```python
from build123d import *

# Parameters (mm, degrees)
BOSS_EXTRUDE1_DEPTH = 35
CUT_EXTRUDE2_DEPTH  = 10
CUT_EXTRUDE3_DEPTH  = 35
SKETCH7_W           = 1.915857316
SKETCH7_H           = 33.660559038
CUT_EXTRUDE4_DEPTH  = 0.1


with BuildPart() as part:
    # Sketch1 → Revolve1 (revolve)
    with BuildSketch(Plane.XY, mode=Mode.PRIVATE) as revolve1_sk:
        Polygon((373.098534333, 35.069747422), (349.598534333, 35.069747422), (349.598534333, 36.051468212), (373.098534333, 36.051468212), (400.761964989, 66.939755158), (401.975618585, 66.939755158), align=None)
    revolve(revolve1_sk.sketch.rotate(Axis((349.598534333, 66.939755158, 0), (0, -1, 0)), 90), axis=Axis((349.598534333, 66.939755158, 0), (0, -1, 0)))

    # Sketch2 → Boss-Extrude1 (add)
    with BuildSketch(Plane(origin=(0, 66.939755158, 0), x_dir=(1, 0, 0), z_dir=(0, 1, 0))):
        with BuildLine():
            ThreePointArc((351.491870795, 51.128386573), (349.575661264, 51.163425543), (347.659483828, 51.12667327))
            Line((347.659483828, 51.12667327), (345.790974227, -51.02155547))
            ThreePointArc((345.790974227, -51.02155547), (347.704525671, -51.128361676), (349.620734741, -51.16342584))
            Line((349.620734741, -51.16342584), (351.491870795, 51.128386573))
        make_face()
    extrude(amount=-BOSS_EXTRUDE1_DEPTH)

    # Sketch3 → Cut-Extrude2 (cut)
    with BuildSketch(Plane(origin=(350.439365404, 0, 6.410285591), x_dir=(0.018289079495206917, 0, -0.9998327407977887), z_dir=(0.9998327407977886, 0, 0.018289079495206913))):
        Polygon((-44.760626875, 65.600314196), (-17.086632512, 35.069747422), (29.874303283, 35.069747422), (57.548297647, 65.600314196), (57.842029456, 31.939755158), (-44.760626875, 31.939755158), align=None)
    extrude(amount=-CUT_EXTRUDE2_DEPTH, mode=Mode.SUBTRACT)

    # Sketch6 → Cut-Extrude3 (cut)
    with BuildSketch(Plane(origin=(0, 66.939755158, 0), x_dir=(1, 0, 0), z_dir=(0, 1, 0))):
        Polygon((350.109498728, -52.374591838), (349.598534333, -52.377084252), (349.598534333, -53.887685529), (342.379231724, -53.887685529), (345.988883028, -52.252553739), align=None)
    extrude(amount=-CUT_EXTRUDE3_DEPTH, mode=Mode.SUBTRACT)


with BuildPart() as cut_extrude3_kept_piece:
    # of the separate pieces the step leaves, the one the design keeps (cut_extrude3_pieces_kept)
    add(part.part.solids().sort_by_distance((350.985738912, 35.069747422, -23.45902094))[0])

    # Sketch7 → Cut-Extrude4 (cut)
    with BuildSketch(Plane(origin=(-0.818630663, 0, 44.753140248), x_dir=(-0.9998327407977887, 0, -0.01828907949520692), z_dir=(0.018289079495206917, 0, -0.9998327407977886))):
        with Locations((-349.540060761, 48.770034677)):
            Rectangle(SKETCH7_W, SKETCH7_H)
    extrude(amount=-CUT_EXTRUDE4_DEPTH, mode=Mode.SUBTRACT)


solid = cut_extrude3_kept_piece.part
```
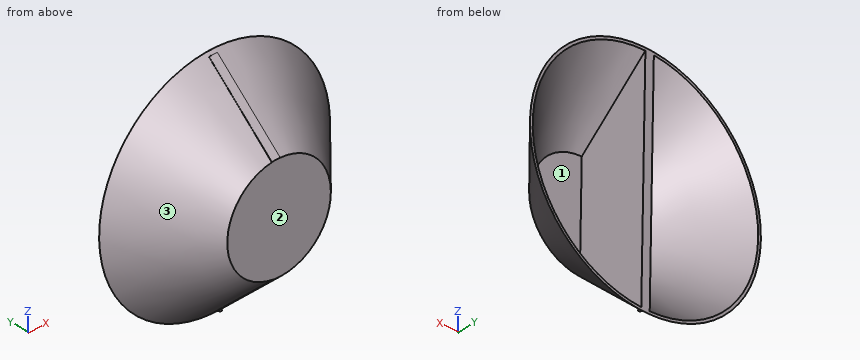
Model file for the job. Use its own axes, mm. Face numbers are marked on the shaded views. Round coordinates to 2 decimals unless told otherwise and drop trailing zeros. Write each loop counter-clockwise with the first axis right and the second up, starting at its lowest first coordinate (ties: lowest second). Pieces come first, ordered by that corner, then holes. Notation, with made-up numbers: (-18, 62.25) - (-8, 62.25) arc R10 cw to (-8, 78.25) - close; hole circle Ø3 at (44, -1.75). An arc over 180 degrees is marked (long way). One line per item, written item: value.
(1) Drop flat-ended pins along their axis: P1, Ø10, axis at x = 374, z = -17, coming from the +Y side; P2, Ø1, axis at x = 378, y = 62, coming from the -Z side; P3, Ø5, axis at x = 372.5, z = 32, coming from the +Y side. Give the stop position or say it passes through.
Values follow:
P1: stops at y = 48.6
P2: stops at z = -39.24
P3: stops at y = 56.54
(2) Cut at B-B, the plane z = 0. Give the cut face in (x, y).
Values follow:
outline: (297.22, 66.94) - (326.1, 35.07) - (373.1, 35.07) - (401.98, 66.94) - (400.76, 66.94) - (373.1, 36.05) - (350.56, 36.05) - (350.56, 66.94) - (346.72, 66.94) - (346.72, 36.05) - (326.1, 36.05) - (298.44, 66.94) - close
(3) Wall check: probe 1 along X at (y, z) = (59.5, 24); probe 2 along X at (y, z) = (38, 6.5); probe 3 along Z at (x, y) = (371, 62.5). Give the ranges that are in metal, low to high.
Values follow:
probe 1: x = 310.78 to 312.12, 346.29 to 350.12, 387.07 to 388.41
probe 2: x = 324.26 to 325.2, 346.61 to 350.44, 373.99 to 374.93
probe 3: z = -43.36 to -42.05, 42.05 to 43.36
(4) Cut at A-A, the plane y = 58. Give the number of separate pieces and of enclosed holes in the cut face, plus the area to 3 significant figures.
Values follow:
separate pieces: 1
enclosed holes: 2
area: 638 mm²
(5) Two-plate mould, pull along Z, no slides. Class the marked faces 1, 2 and 3: pulls with the +Z half, pulls with the -Z half, needs draft (parallel to the pull), parting line crosses it, or undercut.
Values follow:
face 1: undercut
face 2: needs draft
face 3: parting line crosses it
